Here's how the part is built. I have some questions about the finished solid (model axes, mm). Coordinates: 2 decimals unless noted, no trailing zeros. Loops run counter-clockwise (first coordinate to the right, second up) from the corner with the lowest first, then second, coordinate; pieces in that order, holes last.
Autodesk Inventor part; units mm, degrees
ref_plane "Work Plane1" through (8, 0, 0) normal (0, 0, 1) x (1, 0, 0)
ref_plane "YZ Plane" through (0, 0, 0) normal (1, 0, 0) x (0, 1, 0)
ref_plane "XZ Plane" through (0, 0, 0) normal (0, 1, 0) x (-1, 0, 0)
sketch "Skizze1" plane through (0, 0, 0) normal (0, 0, 1) x (1, 0, 0)
  line L0 (0, 0) -> (12.8333, 0)
  line L1 (16, 1.1547) -> (16, 2)
  line L2 (16, 2) -> (0, 2)
  line L3 (16, 1.1547) -> (13.5, 1.1547)
  line L4 (13.5, 1.1547) -> (12.8333, 0)
  line L5 (0, -0.4) -> (0, 2.4)
  line L6 (0, 2) -> (0, 0)
  dimension "d0" = 2.5
  dimension "d1" = 60
  dimension "d2" = 4
  dimension "d3" = 2.3094
  dimension "d5" = 16
revolve "Körper" add sketch "Skizze1" angle 360 about axis through (0, 0, 0) along (1, 0, 0)
sketch "Skizze2" plane through (16, 0, 0) normal (1, 0, 0) x (0, 1, 0)
  circle A0 centre (0, 0) radius 1.1547
  line L0 (-0.5774, 1) -> (0.5774, 1)
  line L1 (0.5774, 1) -> (1.1547, 0)
  line L2 (1.1547, 0) -> (0.5774, -1)
  line L3 (0.5774, -1) -> (-0.5774, -1)
  line L4 (-0.5774, -1) -> (-1.1547, 0)
  line L5 (-1.1547, 0) -> (-0.5774, 1)
  point P0 (0, 0)
  point P1 (0, 0)
extrude "Loch" add sketch "Skizze2" against normal up to next contours L1 A0 | A0 L2 | L0 A0 | A0 L3 | L5 A0 | A0 L4
thread "Gewinde"
chamfer "Fase1" distance 0.4294 angle 45 1 edges at (16, -2, 0) measured on face at (10.6667, 1.9741, -0.3208)
chamfer "Fase2" distance 0.4294 angle 45 1 edges at (0, -2, 0) measured on face at (5.1902, 1.9935, -0.1609)
ref_plane "Work Plane1" through (8, 0, 0) normal (0, 0, 1) x (1, 0, 0)
equation "\"d0\" = INTI"
equation "\"d2\" = NND"
equation "\"d3\" = 1.1547 * SW"
equation "\"d5\" = NLG"
equation "\"d8\" = NLG"
equation "\"d10\" = -0.5 * GD1 + 0.5 * NND"
equation "\"d11\" = FAWI"
equation "\"d34\" = -0.5 * GD1 + 0.5 * NND"
equation "\"d12\" = -0.5 * GD1 + 0.5 * NND"
equation "\"d13\" = FAWI"
equation "\"d35\" = -0.5 * GD1 + 0.5 * NND"
equation "\"NND\" = 4"
equation "\"NLG\" = 16"
equation "\"INTI\" = 2.5"
equation "\"FAWI\" = 45deg"
equation "\"SW\" = 2"
equation "\"GD1\" = THREADDIA - 1.2269 * PTC"
equation "\"SPD\" = 2.5"
equation "\"GUL\" = 0.61345 * PTC"
equation "\"TOA\" = 30deg"
equation "\"THREADDIA\" = 4"
equation "\"PTC\" = 0.7"
equation "\"FAWI1\" = 45deg"
equation "\"GAL\" = 0.61345 * PTC"
equation "\"E0\" = 1.155 * SW"
properties part number "DIN 913 - M4 x 16" material "Stahl, weich"
Q1. Suppose I cut it at A-A on x = 8.5. Write out the boundary of the cut face in (y, z), and give its area (3 significant figures).
Q2. Please list where these lines run through material, in increasing order: probe 1 along X at (y, z) = (0.8, -0.3); probe 2 along X at (y, z) = (-1.7, -0.3); probe 3 along Y at (x, z) = (10.75, -0.55).
Q3. We'd pull the mould along Z, two halves only. Please class faces 1 (the flat face through (0, 0, 0)), 2 (the cylindrical face through (8, 0, 2)), 3 (the flat face through (15, 0, -1)), 4 (the flat face through (14.72, 0.86, 0.51)): pulls with the +Z half, pulls with the -Z half, needs draft (parallel to the pull), parting line crosses it, or undercut.
Check values:
1. outline: circle Ø4 at (0, 0)
1. area: 12.6 mm2
2. probe 1: x = 0 to 13.33
2. probe 2: x = 0.16 to 15.84
2. probe 3: y = -1.92 to 1.92
3. face 1: needs draft
3. face 2: parting line crosses it
3. face 3: undercut
3. face 4: undercut
